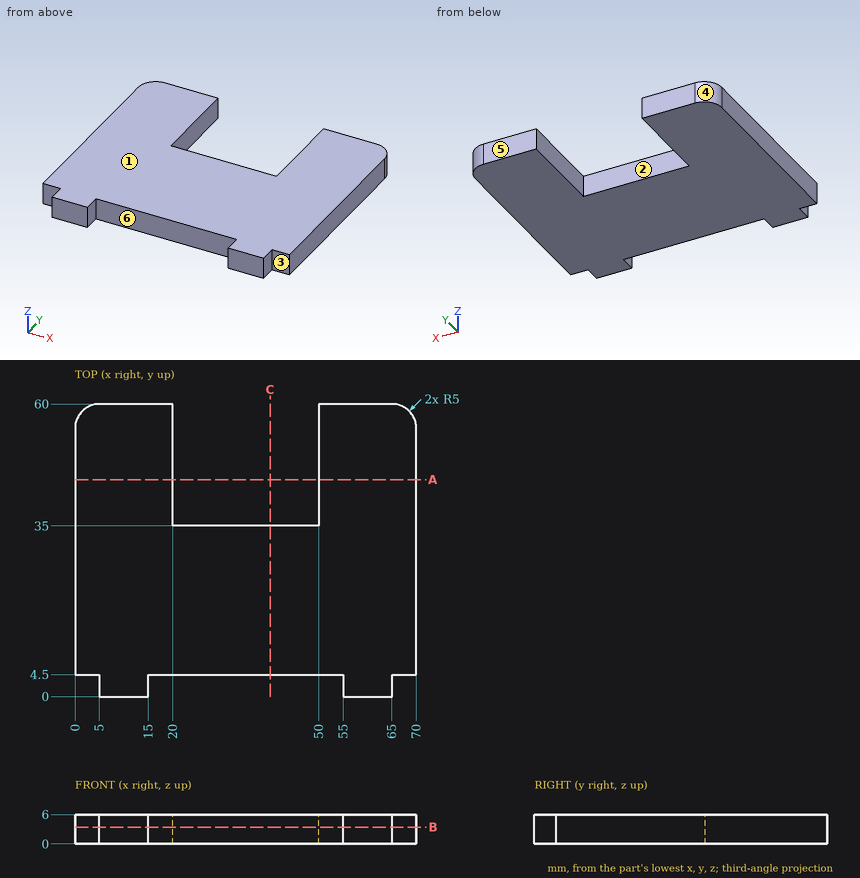
The drawing under review shows one solid part. Ordinate dimensions are in mm from its lowest x, y, z. A direction names the side the tool comes from. Give positions to 0.01 mm unless a question says otherwise; leave off trailing zeros. Order: outer loops, then holes, each group sorted by start corner. A loop starts at its lowest first (then second) coordinate and runs counter-clockwise, first axis right, second up. Notation, with made-up numbers: M -8.5,74.25 L 26.5,74.25 A29 ccw 26.5,95.25 Z; hole C 20,34 d8. An arc over 180 degrees is marked long. Answer in a Markdown table with one row per item. Add a question column.
1. Mouldability with a two-part tool opening along X and no side actions: class the marked faces 4, 5 and 6 as released by +X, released by -X, zero draft, split by the parting line, or undercut.
2. Add section A-A on y = 44.5. State the section outline as (x, z) points.
3. Add section B-B on z = 3.45. State the section outline as (x, y) points.
4. Add section C-C on x = 40. State the section outline as (y, z) points.
5. Machinability: for the marked faces 1, 2 and 3, which of the approach directions +Z, -Z, +X, -X, +Y, -Y give a long, thin tool a straight path to every point of the face, cutting with its end or side? Answer none if there is none.
6. To check wall thickness, follow line 1 along X through (y, z) = (4, 3.1); line 2 along X through (y, z) = (36.5, 5.05); line 3 along Y through (x, z) = (51, 1.8). State the ranges of each line that lie inside material, in increasing order.
7. For pin 1 Ø2.5 at (x, z) = (3, 2) entering from -Y; pin 2 Ø2 at (y, z) = (2.5, 4.5) entering from -X, all flat-tipped, find the tip position at first contact; note any pin that passes through.
The answers:
| question | item | result |
|---|---|---|
| 1 | face 4 | released by -X |
| 1 | face 5 | zero draft |
| 1 | face 6 | undercut |
| 2 | outline | M 0,0 L 20,0 L 20,6 L 0,6 Z; M 50,0 L 70,0 L 70,6 L 50,6 Z |
| 3 | outline | M 0,4.5 L 5,4.5 L 5,0 L 15,0 L 15,4.5 L 55,4.5 L 55,0 L 65,0 L 65,4.5 L 70,4.5 L 70,55 A5 ccw 65,60 L 50,60 L 50,35 L 20,35 L 20,60 L 5,60 A5 ccw 0,55 Z |
| 4 | outline | M 4.5,0 L 35,0 L 35,6 L 4.5,6 Z |
| 5 | face 1 | +Z, +X, -X, +Y, -Y |
| 5 | face 2 | +Z, -Z, +Y |
| 5 | face 3 | +Z, -Z, +X, -Y |
| 6 | line 1 | 5 to 15, 55 to 65 |
| 6 | line 2 | 0 to 20, 50 to 70 |
| 6 | line 3 | 4.5 to 60 |
| 7 | pin 1 | y = 4.5 |
| 7 | pin 2 | x = 5 |
